Here's the drawing with two shaded views (mm, measured from the low corner). I have some questions. Coordinates: 2 decimals unless noted, no trailing zeros. Write each loop counter-clockwise with the first axis right and the second up, starting at its lowest first coordinate (ties: lowest second). Pieces come first, ordered by that corner, then holes. Notation, with made-up numbers: (-24.75, 26.25) - (19.25, 26.25) arc R12 cw to (19.25, 33.25) - close; hole circle Ø3 at (-9, 27.5). An arc over 180 degrees is marked (long way). Answer in a Markdown table with one row per item. Add a question column.
Item 1: I'm going to push a flat-ended pin straight in: pin 1 (3 mm diameter, centred on x = 68, y = 94.5, fed in from -Z). Where does the tip first touch, or does it pass through?
Item 2: Imagine slicing it at B-B (x = 16.5). Please give me the cut outline in (y, z).
Item 3: If I drill on probe 1 along X at (y, z) = (110, 1.5); probe 2 along Y at (x, z) = (18, 1); probe 3 along Z at (x, y) = (19, 92.5), over which ranges is the centre line in solid material (lowest first)? Write a range as from..to.
Item 4: We'd pull the mould along Y, two halves only. Please class the marked faces 1, 2 and 3: +Y half, -Y half, draft (parallel to the pull), parting line (faces both ways), or undercut.
Item 5: Imagine slicing it at A-A (z = 4.5). Please give me the cut outline in (x, y).
Item 6: Imagine slicing it at C-C (y = 72). Please give me the cut outline in (x, z).
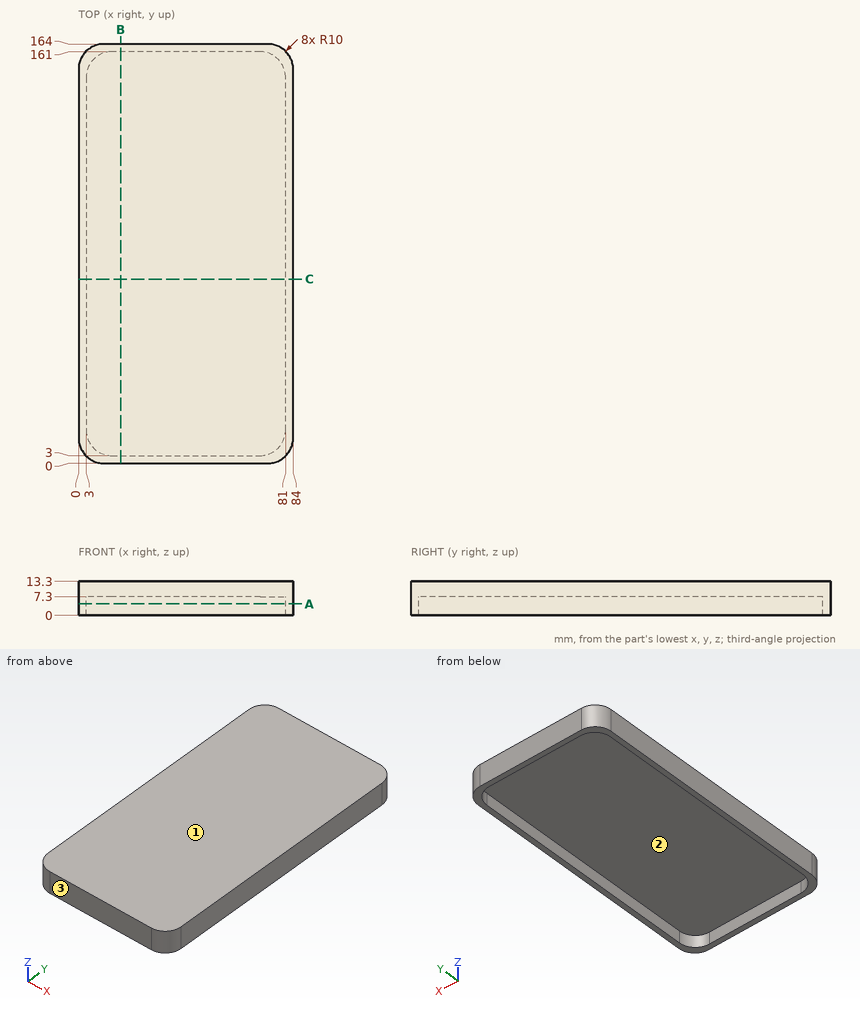
Here are the results:
| question | item | result |
|---|---|---|
| 1 | pin 1 | stops at z = 7.3 |
| 2 | outline | (0, 0) - (3, 0) - (3, 7.3) - (161, 7.3) - (161, 0) - (164, 0) - (164, 13.3) - (0, 13.3) - close |
| 3 | probe 1 | x = 0..3, 81..84 |
| 3 | probe 2 | y = 0..3, 161..164 |
| 3 | probe 3 | z = 7.3..13.3 |
| 4 | face 1 | draft |
| 4 | face 2 | undercut |
| 4 | face 3 | -Y half |
| 5 | outline | (0, 10) arc R10 ccw to (10, 0) - (74, 0) arc R10 ccw to (84, 10) - (84, 154) arc R10 ccw to (74, 164) - (10, 164) arc R10 ccw to (0, 154) - close; hole (3, 13) arc R10 ccw to (13, 3) - (71, 3) arc R10 ccw to (81, 13) - (81, 151) arc R10 ccw to (71, 161) - (13, 161) arc R10 ccw to (3, 151) - close |
| 6 | outline | (0, 0) - (3, 0) - (3, 7.3) - (81, 7.3) - (81, 0) - (84, 0) - (84, 13.3) - (0, 13.3) - close |
